Read the model definition and answer for the solid it produces. Units are mm, in the model's axes. Face numbers are marked on the shaded views. Round coordinates to 2 decimals unless told otherwise and drop trailing zeros. Write each loop counter-clockwise with the first axis right and the second up, starting at its lowest first coordinate (ties: lowest second). Pieces come first, ordered by that corner, then holes. Notation, with made-up numbers: (-15, 24.5) - (14, 24.5) arc R22 ccw to (14, 42.5) - close; hole circle Ø10 at (89, 89.25). An arc over 180 degrees is marked (long way). One line per item, written item: value. Start each with the question number.
(1) Flat-ended cylindrical pins translate along their axes: pin 1 Ø2 at (y, z) = (0, 5.5) entering from -X; pin 2 Ø1 at (x, z) = (1, 1.5) entering from +Y; pin 3 Ø3 at (x, y) = (0, 0) entering from -Z; pin 4 Ø1 at (y, z) = (-1, 7) entering from +X. Find the tip coordinate at first contact, or state that the pin passes through.
(2) The mould has two halves that part along Y. Classify the marked faces 1, 2 and 3: +Y half, -Y half, draft (parallel to the pull), parting line (faces both ways), or undercut.
(3) Find the intervals of material crossed by L1, parallel to Y at x = 0, z = 3.5; L2, parallel to Z at x = 1.25, y = 2.1; L3, parallel to X at y = 0.45, z = 1.5, in increasing order.
(4) A cutting plane is placed at C-C, the plane z = 4.5. Determine the outline of the cut face in (x, y).
(5) A cutting plane is placed at D-D, the plane x = -2.4. Determine the outline of the cut face in (y, z), plus the area to 3 significant figures.
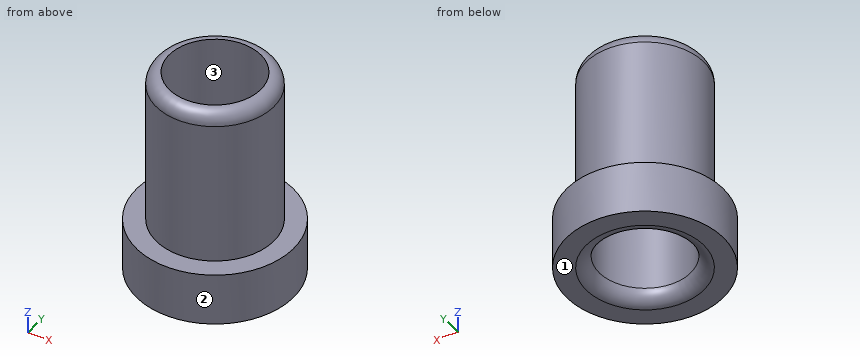
from build123d import *

# Parameters (mm, degrees)
F0_R     = 3
F0_R_2   = 2.25
F1_DEPTH = 2
F0_R_3   = 1.75
F2_DEPTH = 8
F3_R     = 0.5
F4_R     = 0.49999


# Not quite as in the source:
# - a fillet or chamfer is up to 0.001 mm smaller than in the source, because OpenCascade refuses the exact size


with BuildPart() as f1:
    # F0 (on Top) → F1 (new body)
    with BuildSketch(Plane.XY):
        Circle(F0_R)
        Circle(F0_R_2, mode=Mode.SUBTRACT)
    extrude(amount=F1_DEPTH)

    # F0 (on Top) → F2 (join)
    with BuildSketch(Plane.XY):
        Circle(F0_R_2)
        Circle(F0_R_3, mode=Mode.SUBTRACT)
    extrude(amount=F2_DEPTH)

    # F3
    f3_edges = [f1.edges().sort_by_distance(p)[0] for p in [
        (-1.75, 0, 0),
    ]]
    fillet(f3_edges, radius=F3_R)

    # F4 (radius 0.5 in the source; OpenCascade refuses exactly that, so slightly less here)
    f4_edges = [f1.edges().sort_by_distance(p)[0] for p in [
        (-2.25, 0, 8),
    ]]
    fillet(f4_edges, radius=F4_R)


solid = f1.part
Here are the results:
1. pin 1: x = -2.25
1. pin 2: y = 2.96
1. pin 3: through
1. pin 4: x = 2.19
2. face 1: draft
2. face 2: parting line
2. face 3: undercut
3. L1: -2.25 to -1.75, 1.75 to 2.25
3. L2: 0 to 2
3. L3: -2.97 to -1.69, 1.69 to 2.97
4. outline: circle Ø4.5 at (0, 0); hole circle Ø3.5 at (0, 0)
5. outline: (-1.8, 0) - (1.8, 0) - (1.8, 2) - (-1.8, 2) - close
5. area: 7.20 mm²
